```python
from build123d import *

# Parameters (mm, degrees)
SKETCH1_W           = 63
SKETCH1_H           = 63
SKETCH1_R           = 2.5
BOSS_EXTRUDE1_DEPTH = 1.5
SKETCH2_R           = 25
BOSS_EXTRUDE2_DEPTH = 80
CHAMFER1_SIZE       = 10
CHAMFER1_SIZE2      = 1.943803091


with BuildPart() as part:
    # Sketch1 → Boss-Extrude1 (new body)
    with BuildSketch(Plane.XY):
        Rectangle(SKETCH1_W, SKETCH1_H)
        with Locations((24, 24)):
            Circle(SKETCH1_R, mode=Mode.SUBTRACT)
        with Locations((24, -24)):
            Circle(SKETCH1_R, mode=Mode.SUBTRACT)
        with Locations((-24, -24)):
            Circle(SKETCH1_R, mode=Mode.SUBTRACT)
        with Locations((-24, 24)):
            Circle(SKETCH1_R, mode=Mode.SUBTRACT)
    extrude(amount=BOSS_EXTRUDE1_DEPTH)

    # Sketch2 → Boss-Extrude2 (add)
    with BuildSketch(Plane.XY.offset(1.5)):
        Circle(SKETCH2_R)
    extrude(amount=BOSS_EXTRUDE2_DEPTH)

    # Chamfer1
    chamfer1_edges = [part.edges().sort_by_distance(p)[0] for p in [
        (-25, 0, 81.5),
    ]]
    chamfer1_side = [part.faces().sort_by_distance(p)[0] for p in [
        (-25, 0, 41.5),
    ]]
    chamfer(chamfer1_edges, length=CHAMFER1_SIZE, length2=CHAMFER1_SIZE2, reference=chamfer1_side[0])


solid = part.part
```
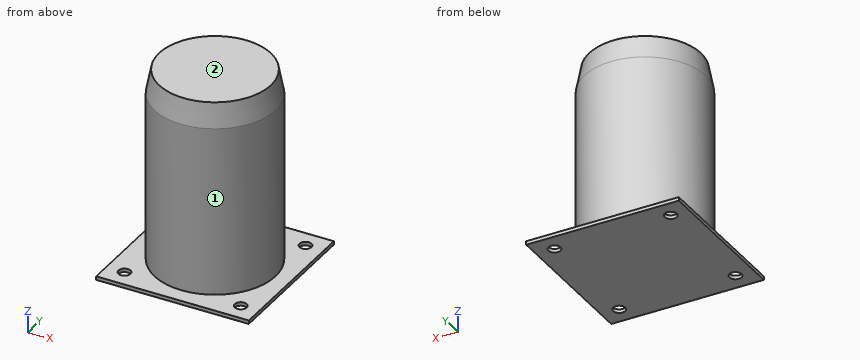
Check sheet for the modelled part. Datum: model origin and axes. Units: mm. Face numbers are marked on the shaded views. A direction names the side the tool comes from. Give positions to 0.01 mm unless a question says otherwise; leave off trailing zeros. Write each loop counter-clockwise with the first axis right and the second up, starting at its lowest first coordinate (ties: lowest second). Pieces come first, ordered by that corner, then holes. Notation, with made-up numbers: (52, -1) - (102, -1) arc R21 cw to (102, 15) - close; hole circle Ø6 at (71.25, 48). An arc over 180 degrees is marked (long way). Answer as a JSON object with one key per item and string values. Group by question number.
1) Sectioned sample at A-A (x = 0). Record the cut outline in (y, z), then the cut area to 3 significant figures.
2) Access from +Z, -Z, +X, -X, +Y, -Y to the whole of each face (thin tool, end or side, straight path). Record for the marked faces 1 and 2.
3) Sectioned sample at B-B (z = 16). Record the cut outline in (x, y), then the cut area to 3 significant figures.
4) Thickness scan on probe 1 along Y at (x, z) = (-24, 1.15); probe 2 along Z at (x, y) = (26, 28.5); probe 3 along Y at (x, z) = (1, 63). Record the ranges inside material, lowest first. Write a range as from..to.
5) Depth check by flat-ended pin: P1, Ø8, axis at x = 22, z = 60, coming from the -Y side; P2, Ø8, axis at y = 15.5, z = 11, coming from the -X side; P3, Ø1.5, axis at x = 21.5, z = 45.5, coming from the +Y side; P4, Ø3, axis at x = -24, y = -24, coming from the -Z side. Enter the tip coordinate at first touch or a pass-through.
Geometry results:
{
 "1": {"outline": "(-31.5, 0) - (31.5, 0) - (31.5, 1.5) - (25, 1.5) - (25, 71.5) - (23.06, 81.5) - (-23.06, 81.5) - (-25, 71.5) - (-25, 1.5) - (-31.5, 1.5) - close", "area": "4,080 mm^2"},
 "2": {"face 1": "+Z", "face 2": "+Z, +X, -X, +Y, -Y"},
 "3": {"outline": "circle Ø50 at (0, 0)", "area": "1,960 mm^2"},
 "4": {"probe 1": "y = -31.5..-26.5, -21.5..21.5, 26.5..31.5", "probe 2": "z = 0..1.5", "probe 3": "y = -24.98..24.98"},
 "5": {"P1": "stops at y = -17.35", "P2": "stops at x = -22.2", "P3": "stops at y = 13.94", "P4": "passes through"}
}
